```python
from build123d import *

# Parameters (mm, degrees)
BOSS_EXTRUDE1_DEPTH                     = 14
FILLET1_R                               = 1
CBORE_FOR_M5_HEX_HEAD_BOLT1_D           = 4
CBORE_FOR_M5_HEX_HEAD_BOLT1_DEPTH       = 8
CBORE_FOR_M5_HEX_HEAD_BOLT1_CBORE_D     = 7
CBORE_FOR_M5_HEX_HEAD_BOLT1_CBORE_DEPTH = 4.5
M5_TAPPED_HOLE1_D                       = 3.5
M5_TAPPED_HOLE1_DEPTH                   = 8
M5_TAPPED_HOLE1_CSINK_D                 = 5.5
M5_TAPPED_HOLE1_CSINK_ANGLE             = 90
CHAMFER1_SIZE                           = 0.5


with BuildPart() as part:
    # Sketch1 → Boss-Extrude1 (new body)
    with BuildSketch(Plane.XY):
        with BuildLine():
            Line((-21, -20), (21, -20))
            Line((21, -20), (21, -13.3))
            Line((21, -13.3), (9, -13.3))
            Line((9, -13.3), (9, 13.4))
            Line((9, 13.4), (1, 13.4))
            Line((1, 13.4), (1, 3.872983346))
            ThreePointArc((1, 3.872983346), (0, -4), (-1, 3.872983346))
            Line((-1, 3.872983346), (-1, 13.4))
            Line((-1, 13.4), (-9, 13.4))
            Line((-9, 13.4), (-9, -13.3))
            Line((-9, -13.3), (-21, -13.3))
            Line((-21, -13.3), (-21, -20))
        make_face()
    extrude(amount=BOSS_EXTRUDE1_DEPTH)

    # Fillet1
    fillet1_edges = [part.edges().sort_by_distance(p)[0] for p in [
        (-21, -13.3, 7),
        (-9, -13.3, 7),
        (-9, 13.4, 7),
        (9, 13.4, 7),
        (9, -13.3, 7),
        (21, -13.3, 7),
        (21, -20, 7),
        (-21, -20, 7),
    ]]
    fillet(fillet1_edges, radius=FILLET1_R)

    # CBORE for M5 Hex Head Bolt1
    with Locations(Plane(origin=(9, 0, 0), x_dir=(0, 0, -1), z_dir=(1, 0, 0))):
        with Locations((-7, 8.2)):
            CounterBoreHole(CBORE_FOR_M5_HEX_HEAD_BOLT1_D / 2, CBORE_FOR_M5_HEX_HEAD_BOLT1_CBORE_D / 2, CBORE_FOR_M5_HEX_HEAD_BOLT1_CBORE_DEPTH, depth=CBORE_FOR_M5_HEX_HEAD_BOLT1_DEPTH)

    # M5 Tapped Hole1
    with Locations(Plane.ZY.offset(9)):
        with Locations((7, 8.2)):
            CounterSinkHole(M5_TAPPED_HOLE1_D / 2, M5_TAPPED_HOLE1_CSINK_D / 2, depth=M5_TAPPED_HOLE1_DEPTH, counter_sink_angle=M5_TAPPED_HOLE1_CSINK_ANGLE)

    # Sketch8 → CSK for M5 Countersunk Flat Head Screw2 (revolve, cut)
    with BuildSketch(Plane(origin=(16.25, -13.3, 7), x_dir=(0, 0, 1), z_dir=(1, 0, 0))):
        Polygon((0, 0), (0, 6.7), (3.5, 6.7), (2.75, 5.95), (2.75, 0.75), (3.5, 0), align=None)
    revolve(axis=Axis((16.25, -6.95, 7), (0, -1, 0)), mode=Mode.SUBTRACT)

    # Sketch10 → CSK for M5 Countersunk Flat Head Screw3 (revolve, cut)
    with BuildSketch(Plane(origin=(-16.25, -13.3, 7), x_dir=(0, 0, 1), z_dir=(1, 0, 0))):
        Polygon((0, 0), (0, 6.7), (3.5, 6.7), (2.75, 5.95), (2.75, 0.75), (3.5, 0), align=None)
    revolve(axis=Axis((-16.25, -6.95, 7), (0, -1, 0)), mode=Mode.SUBTRACT)

    # Chamfer1
    chamfer1_edges = [part.edges().sort_by_distance(p)[0] for p in [
        (0, -4, 0),
        (0, -4, 14),
    ]]
    chamfer(chamfer1_edges, length=CHAMFER1_SIZE)


solid = part.part
```
For this review, take the finished solid that the model builds, in its own axes (mm). A direction names the side the tool comes from. Round coordinates to 2 decimals unless told otherwise and drop trailing zeros. Write each loop counter-clockwise with the first axis right and the second up, starting at its lowest first coordinate (ties: lowest second). Pieces come first, ordered by that corner, then holes. Notation, with made-up numbers: M 51.5,65.25 L 75.5,65.25 A16 cw 75.5,92.25 Z; hole C 48.25,58 d2. An arc over 180 degrees is marked long. One line per item, written item: value. Start each with the question number.
(1) Wall thickness on line 1 (X direction, y = -17.6, z = 7); line 2 (X direction, y = 0, z = 8.5); line 3 (Y direction, x = -4.5, z = 7): over which ranges is each line inside the solid? List them lowest first.
(2) We need section A-A (x = 16.25). Give the boundary of the cut face in (y, z), and give its area (3 significant figures).
(3) The part is to be moulded in two halves that separate along Y. For faces 1 (the cylindrical face through (-19, -17, 7)), 2 (the flat face through (-13, -13.3, 5)), 3 (the conical face through (0.169, -4.132, 0.365)), say which applies: released by +Y, released by -Y, zero draft, split by the parting line, or undercut.
(4) Machinability: for faces 4 (the flat face through (21, -17, 7)), 5 (the flat face through (1, 9.8, 8.5)), which of the approach directions +Z, -Z, +X, -X, +Y, -Y give a long, thin tool a straight path to every point of the face, cutting with its end or side? Answer none if there is none.
(5) We need section B-B (y = 0). Give the boundary of the cut face in (x, z).
(6) Insertion check: pin 1 (2 mm diameter, centred on x = 5.5, y = -14, fed in from -Z); pin 2 (6.5 mm diameter, centred on y = 8.2, z = 7, fed in from -X); pin 3 (3 mm diameter, centred on x = -13.5, z = 9.5, fed in from +Y); pin 4 (4.5 mm diameter, centred on y = 8.2, z = 7, fed in from +X). Each pin has a flat end and moves straight along its axis. Give the tip position at first contact, or say it passes through.
(7) We need section D-D (y = 8.2). Give the boundary of the cut face in (x, z).
(8) We need section C-C (z = 1.5). Give the boundary of the cut face in (x, y).
Result:
1. line 1: -21 to -19, -13.5 to 13.5, 19 to 21
1. line 2: -9 to -4, 4 to 9
1. line 3: -20 to 6.45, 9.95 to 13.4
2. outline: M -20,0 L -13.3,0 L -13.3,3.5 L -14.05,4.25 L -19.25,4.25 L -20,3.5 Z; M -20,10.5 L -19.25,9.75 L -14.05,9.75 L -13.3,10.5 L -13.3,14 L -20,14 Z
2. area: 55.8 mm²
3. face 1: zero draft
3. face 2: released by +Y
3. face 3: undercut
4. face 4: +Z, -Z, +X, +Y, -Y
4. face 5: +Z, -Z, +Y
5. outline: M -9,0 L -4.5,0 L -4,0.5 L -4,13.5 L -4.5,14 L -9,14 Z; M 4,0.5 L 4.5,0 L 9,0 L 9,14 L 4.5,14 L 4,13.5 Z
6. pin 1: z = 0
6. pin 2: x = -9
6. pin 3: y = -13.3
6. pin 4: x = 4.5
7. outline: M -9,0 L -1,0 L -1,5.25 L -8,5.25 L -9,4.25 Z; M -9,9.75 L -8,8.75 L -1,8.75 L -1,14 L -9,14 Z; M 1,0 L 9,0 L 9,3.5 L 4.5,3.5 L 4.5,5 L 1,5 Z; M 1,9 L 4.5,9 L 4.5,10.5 L 9,10.5 L 9,14 L 1,14 Z
8. outline: M -21,-19 A1 ccw -20,-20 L 20,-20 A1 ccw 21,-19 L 21,-14.3 A1 ccw 20,-13.3 L 10,-13.3 A1 cw 9,-12.3 L 9,12.4 A1 ccw 8,13.4 L 1,13.4 L 1,3.87 A4 cw long -1,3.87 L -1,13.4 L -8,13.4 A1 ccw -9,12.4 L -9,-12.3 A1 cw -10,-13.3 L -20,-13.3 A1 ccw -21,-14.3 Z
